Input: part model. Units: mm. Frame: model coordinates. Round coordinates to 2 decimals unless told otherwise and drop trailing zeros. Write each loop counter-clockwise with the first axis right and the second up, starting at its lowest first coordinate (ties: lowest second). Pieces come first, ordered by that corner, then holes. Notation, with made-up numbers: (82.5, 88) -> (129.5, 88) arc R18 cw to (129.5, 103) -> close; hole circle Ø6 at (-4, 1). An arc over 180 degrees is marked (long way). Use CSV: the item, a comma, the result in double quotes.
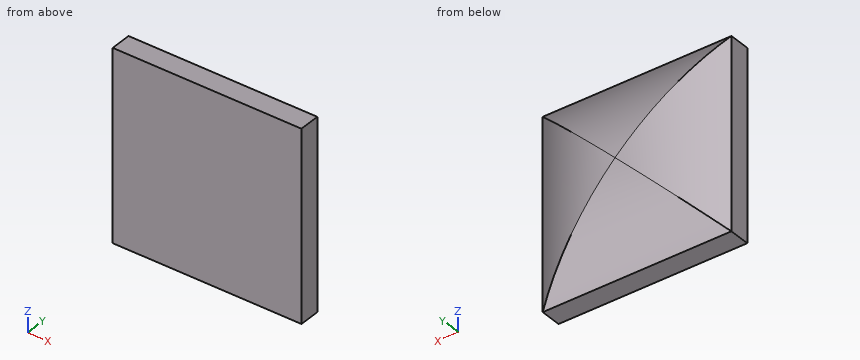
```python
from build123d import *

# Parameters (mm, degrees)
BOSS_EXTRUDE6_DEPTH = 45
BOSS_EXTRUDE8_DEPTH = 45


with BuildPart() as part:
    # Sketch4 → Boss-Extrude6 (new, symmetric)
    with BuildSketch(Plane.XY):
        with BuildLine():
            Line((-45, 0), (45, 0))
            Line((45, 0), (45, 10))
            ThreePointArc((45, 10), (0, 23.856217223), (-45, 10))
            Line((-45, 10), (-45, 0))
        make_face()
    extrude(amount=BOSS_EXTRUDE6_DEPTH, both=True)


with BuildPart() as body_2:
    # Sketch9 → Boss-Extrude8 (new, symmetric)
    with BuildSketch(Plane(origin=(0, 0, 0), x_dir=(0, 0, -1), z_dir=(1, 0, 0))):
        with BuildLine():
            Line((-45, 0), (45, 0))
            Line((45, 0), (45, 10))
            ThreePointArc((45, 10), (0, 23.856217223), (-45, 10))
            Line((-45, 10), (-45, 0))
        make_face()
    extrude(amount=BOSS_EXTRUDE8_DEPTH, both=True)


with BuildPart() as part_1:
    add(part.part)

    # Combine1: intersect body 2
    add(body_2.part, mode=Mode.INTERSECT)


solid = part_1.part
```
Item 1: Line query: line 1 (Y direction, x = 31, z = -0.5); line 2 (Z direction, x = -28, y = 13.5); line 3 (Y direction, x = -23.5, z = -39). Output: solid intervals per line, ascending.
Worked answers:
line 1,"y = 0 to 17.61"
line 2,"z = -39.37 to 39.37"
line 3,"y = 0 to 13.71"
Item 2: First-contact query: pin 1 Ø8 at (y, z) = (15, 23.5) entering from -X; pin 2 Ø3 at (x, y) = (-27.5, 18) entering from +Z. Flat tips, straight axial feed; report the tip coordinate or a pass-through.
Worked answers:
pin 1,"stops at x = -43.49"
pin 2,"stops at z = 33.51"
Item 3: Section query A-A on z = 2.5. Return the cut outline in (x, y), plus the area to 3 significant figures.
Worked answers:
outline,"(-45, 0) -> (45, 0) -> (45, 10) arc R80 ccw to (2.5, 23.82) -> (-2.5, 23.82) arc R80 ccw to (-45, 10) -> close"
area,"1,750 mm²"
Item 4: Section query C-C on y = 15.75. Return the cut outline in (x, z).
Worked answers:
outline,"(-35.09, -35.09) -> (35.09, -35.09) -> (35.09, 35.09) -> (-35.09, 35.09) -> close"
Item 5: Section query B-B on x = -38. Return the cut outline in (y, z).
Worked answers:
outline,"(0, -45) -> (10, -45) arc R80 ccw to (14.26, -38) -> (14.26, 38) arc R80 ccw to (10, 45) -> (0, 45) -> close"
